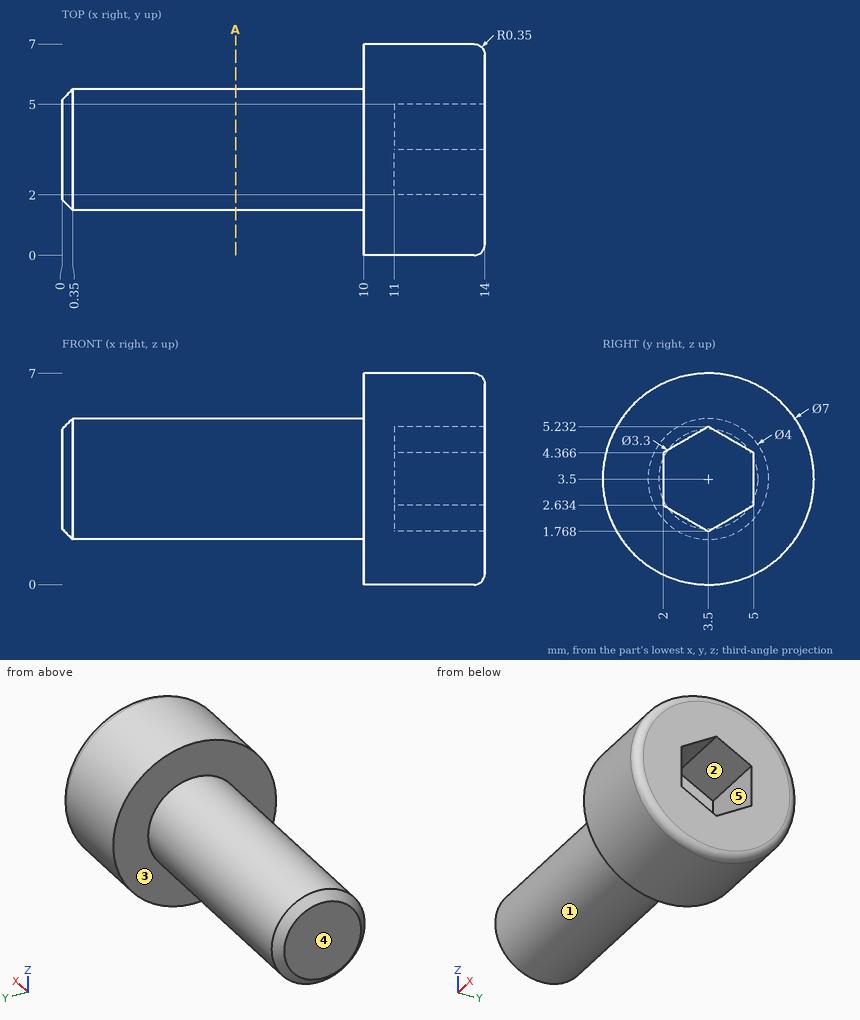
Geometry check sheet. Reference: drawing and pictorial views, mm from the part's lowest x, y, z. A direction names the side the tool comes from. Coordinates: 2 decimals unless noted, no trailing zeros. Write each loop counter-clockwise with the first axis right and the second up, starting at its lowest first coordinate (ties: lowest second). Pieces come first, ordered by that corner, then holes. Notation, with made-up numbers: M -12,-36.5 L -5,-36.5 A8 ccw -5,-23.5 Z; hole C 7.25,-17.75 d5. An arc over 180 degrees is marked long. Use one line per item in the form item = value.
Item 1: Set-up check for the marked faces 4 and 5: record each of +Z, -Z, +X, -X, +Y, -Y from which the full face is reachable in a straight line by a thin tool's end or side.
Answer below:
face_4 = +Z, -Z, -X, +Y, -Y
face_5 = +X
Item 2: Sectioned sample at A-A, the plane x = 5.75. Record the cut outline in (y, z).
Answer below:
outline = C 3.5,3.5 d4
Item 3: Gauge pin test, flat ends, axial feed: pin 1 Ø1.5 at (y, z) = (2, 5) entering from -X; pin 2 Ø4 at (x, z) = (4.5, 1.5) entering from -Y; pin 3 Ø0.9 at (y, z) = (4, 3.5) entering from +X. Record the tip position at first contact, or that the pin passes through.
Answer below:
pin_1 = 0
pin_2 = 1.5
pin_3 = 11
Item 4: Release check for a two-part mould opening along Z. For the marked faces 1, 2 and 3 record: pulls with the +Z half, pulls with the -Z half, needs draft (parallel to the pull), parting line crosses it, or undercut.
Answer below:
face_1 = parting line crosses it
face_2 = undercut
face_3 = needs draft
Item 5: Material ranges on L1, parallel to X at y = 4, z = 6.25; L2, parallel to Y at x = 2.25, z = 2.5, recorded low to high. Write a range as from..to.
Answer below:
L1 = 10..14
L2 = 1.77..5.23
